Can you work these out from the model? Positions are in its coordinate system, mm. A direction names the side the tool comes from. Give positions to 0.01 mm unless a question says otherwise; leave off trailing zeros. Loops run counter-clockwise (first coordinate to the right, second up) from the corner with the lowest first, then second, coordinate; pieces in that order, holes last. Notation, with made-up numbers: (-19, 82) - (0, 82) arc R16 ccw to (0, 110) - close; hole circle Ø10 at (56, 32). An arc over 180 degrees is marked (long way). Answer as a JSON object with one key per item and string values. Group by question number.
Item 1: Suppose I cut it at A-A on z = -63. Write out the boundary of the cut face in (x, y), and give its area (3 significant figures).
Item 2: Will these pins go through, and if not, where does the flat tip stop? pin 1 (2 mm diameter, centred on y = -3.5, z = -11.5, fed in from -X); pin 2 (1.5 mm diameter, centred on y = -3, z = 24, fed in from +X); pin 3 (13 mm diameter, centred on x = 20, z = 45, fed in from +Y); pin 4 (4 mm diameter, centred on x = 63, y = -2.5, fed in from +Z).
Item 3: Suppose I cut it at C-C on z = 45. Write out the boundary of the cut face in (x, y).
Item 4: Please list where these lines run through material, in increasing order: L1, parallel to X at y = -5.25, z = 45; L2, parallel to X at y = -3.25, z = 82; L3, parallel to Y at x = -35.5, z = 27.
Item 5: Suppose I cut it at B-B on x = 0. Write out the boundary of the cut face in (y, z).
Item 6: Which directions (+Z, -Z, +X, -X, +Y, -Y) give clear straight access to the entire face, cutting with the end or side of a thin tool? Please do faces 1 (the cylindrical face through (66.014, -2.958, -119.297)), 2 (the cylindrical face through (-23.76, -2.96, 121.44)), 3 (the flat face through (-45, -3, 64)).
Item 7: Suppose I cut it at D-D on y = -1.25. Count the separate pieces of the cut face and the enclosed holes in it, and give its area (3 significant figures).
Item 8: Thinking about a two-plate mould opening in Z: for faces 4 (the flat face through (1, 0, -2)), 5 (the cylindrical face through (-17.3, -3.55, 47.95)), 6 (the flat face through (-69.5, -3.04, -9.41)), which applies, pulls with the +Z half, pulls with the -Z half, needs draft (parallel to the pull), parting line crosses it, or undercut?
Solid Edge part; units mm, degrees
sketch "Sketch1" plane through (0, 0, 0) normal (0, -1, 0) x (1, 0, 0)
  line L0 (-100, 125) -> (100, 125)
  line L1 (100, 125) -> (100, -125)
  line L2 (100, -125) -> (-100, -125)
  line L3 (-100, -125) -> (-100, 125)
  dimension "D1" = 100
  dimension "D2" = 100
extrude "Protrusion1" add sketch "Sketch1" along normal blind 6
sketch "Sketch2" plane through (0, -6, 0) normal (0, -1, 0) x (1, 0, 0)
  line L0 (-30, 55) -> (30, 55)
  line L1 (30, 55) -> (30, -5)
  line L2 (30, -5) -> (-30, -5)
  line L3 (-30, -5) -> (-30, 55)
  dimension "D1" = 30
  dimension "D2" = 30
extrude "Ausprägung_2" add sketch "Sketch2" along normal blind 1
sketch "Sketch3" plane through (0, -6, 0) normal (0, -1, 0) x (1, 0, 0)
  line L0 (-60, -45) -> (60, -45)
  line L1 (60, -45) -> (60, -125)
  line L2 (60, -125) -> (-60, -125)
  line L3 (-60, -125) -> (-60, -45)
  dimension "D1" = 60
extrude "Ausschnitt_1" cut sketch "Sketch3" against normal blind 66.675
sketch "Sketch4" plane through (0, -6, 0) normal (0, -1, 0) x (1, 0, 0)
  line L0 (-20, 125) -> (20, 125)
  line L1 (20, 125) -> (20, 75)
  line L2 (20, 75) -> (-20, 75)
  line L3 (-20, 75) -> (-20, 125)
  dimension "D1" = 20
  dimension "D2" = 20
extrude "Ausschnitt_2" cut sketch "Sketch4" against normal blind 63.5
sketch "Sketch5" plane through (0, -6, 0) normal (0, -1, 0) x (1, 0, 0)
  line L0 (-45, 125) -> (-45, 11.1505)
  line L1 (-45, 11.1505) -> (-100, -35)
  line L2 (-100, -35) -> (-100, 125)
  line L3 (-100, 125) -> (-45, 125)
  dimension "D1" = 100
extrude "Ausschnitt_3" cut sketch "Sketch5" against normal blind 66.675
sketch "Sketch6" plane through (0, -6, 0) normal (0, -1, 0) x (1, 0, 0)
  line L0 (45, 125) -> (45, 11.1505)
  line L1 (45, 11.1505) -> (100, -35)
  line L2 (100, -35) -> (100, 125)
  line L3 (100, 125) -> (45, 125)
  dimension "D1" = 100
extrude "Ausschnitt_4" cut sketch "Sketch6" against normal blind 117.475
sketch "Sketch7" plane through (0, 0, 0) normal (0, 1, 0) x (-1, 0, 0)
  circle A0 centre (0, -12) radius 5
  circle A1 centre (0, 62) radius 5
extrude "Ausschnitt_7" cut sketch "Sketch7" against normal blind 127
sketch "Sketch8" plane through (0, -6, 0) normal (0, -1, 0) x (1, 0, 0)
  line L0 (-20, 75) -> (-3.5431, 58.4721)
  line L1 (-3.5431, 58.4721) -> (3.5431, 58.4721)
  line L2 (3.5431, 58.4721) -> (20, 75)
  line L3 (20, 75) -> (-20, 75)
extrude "Ausschnitt_8" cut sketch "Sketch8" against normal blind 400.05
sketch "Sketch9" plane through (0, -6, 0) normal (0, -1, 0) x (1, 0, 0)
  line L0 (-60, -45) -> (-2.7231, -7.8066)
  line L1 (-2.7231, -7.8066) -> (2.7231, -7.8066)
  line L2 (2.7231, -7.8066) -> (60, -45)
  line L3 (60, -45) -> (-60, -45)
extrude "Ausschnitt_9" cut sketch "Sketch9" against normal blind 565.15
hole "Bohrung_4" at (20, -7, 45) direction (0, 1, 0) diameter 8 end up to next
hole "Hole1" at (0, -7, 5) direction (0, 1, 0) diameter 8 end up to next
hole "Hole2" at (-20, -7, 45) direction (0, 1, 0) diameter 8 end up to next
fillet "Verrundung_1" radius 5 6 edges at (-45, -3, 11.1505) (-20, -3, 75) (20, -3, 75) (45, -3, 11.1505) (60, -3, -45) (-60, -3, -45)
fillet "Verrundung_2" radius 12.5 4 edges at (-45, -3, 125) (-20, -3, 125) (20, -3, 125) (45, -3, 125)
fillet "Verrundung_3" radius 20 1 edges at (-100, -3, -35)
fillet "Verrundung_4" radius 20 1 edges at (100, -3, -35)
fillet "Verrundung_5" radius 20 4 edges at (-100, -3, -125) (-60, -3, -125) (60, -3, -125) (100, -3, -125)
properties material "Aluminium, 1060"
Worked out:
{
 "1": {"outline": "(-100, -6) - (-60, -6) - (-60, 0) - (-100, 0) - close; (60, -6) - (100, -6) - (100, 0) - (60, 0) - close", "area": "480 mm2"},
 "2": {"pin 1": "stops at x = -73.19", "pin 2": "stops at x = 45", "pin 3": "stops at y = 0", "pin 4": "stops at z = -2.28"},
 "3": {"outline": "(-45, -6) - (-30, -6) - (-30, -7) - (-24, -7) - (-24, 0) - (-45, 0) - close; (-16, -7) - (16, -7) - (16, 0) - (-16, 0) - close; (24, -7) - (30, -7) - (30, -6) - (45, -6) - (45, 0) - (24, 0) - close"},
 "4": {"L1": "x = -45 to -24, -16 to 16, 24 to 45", "L2": "x = -45 to -20, 20 to 45", "L3": "y = -6 to 0"},
 "5": {"outline": "(-7, -5) - (-6, -5) - (-6, -7) - (0, -7) - (0, 1) - (-7, 1) - close; (-7, 9) - (0, 9) - (0, 57) - (-6, 57) - (-6, 55) - (-7, 55) - close"},
 "6": {"face 1": "-Z, +Y, -Y", "face 2": "+Z, +Y, -Y", "face 3": "+Z, -X, +Y, -Y"},
 "7": {"separate pieces": "1", "enclosed holes": "3", "area": "20,000 mm2"},
 "8": {"face 4": "needs draft", "face 5": "undercut", "face 6": "pulls with the +Z half"}
}
